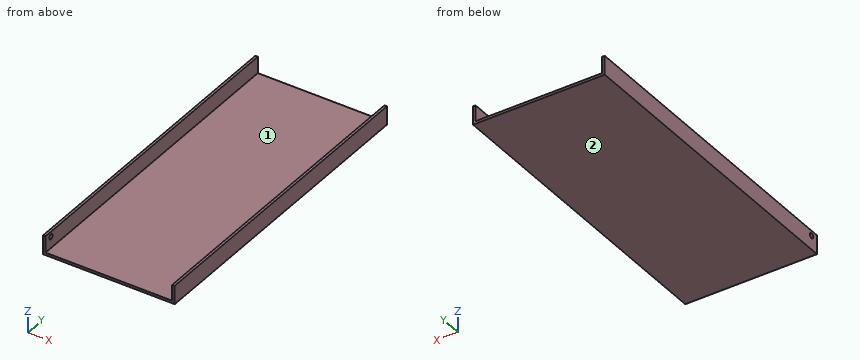
```python
from build123d import *

# Parameters (mm, degrees)
F1_DEPTH = 500
F3_D     = 8
F3_DEPTH = 12


with BuildPart() as f1:
    # F0 (on Front) → F1 (new body)
    with BuildSketch(Plane.XZ):
        Polygon((-104, 30), (-104, 0), (104, 0), (104, 29.331477), (100, 29.331477), (100, 4), (-100, 4), (-100, 30), align=None)
    extrude(amount=-F1_DEPTH)

    # F3
    with Locations(Plane(origin=(-104, 0, 0), x_dir=(0, -1, 0), z_dir=(-1, 0, 0))):
        with Locations((-12.759611, 22.157129)):
            Hole(F3_D / 2, depth=F3_DEPTH)


solid = f1.part
```
Geometry check sheet. Reference: the model listing, model coordinates, mm. Face numbers are marked on the shaded views. Coordinates: 2 decimals unless noted, no trailing zeros. Loops run counter-clockwise (first coordinate to the right, second up) from the corner with the lowest first, then second, coordinate; pieces in that order, holes last.
Item 1: Thickness scan on line 1 (X direction, y = 106, z = 25); line 2 (Z direction, x = -19, y = 406.5). Record the ranges inside material, lowest first.
Item 2: Sectioned sample at C-C, the plane x = 53. Record the boundary of the cut face in (y, z).
Item 3: Release check for a two-part mould opening along X. For the marked faces 1 and 2 record: released by +X, released by -X, zero draft, split by the parting line, or undercut.
Item 4: Sectioned sample at B-B, the plane y = 225.5. Record the boundary of the cut face in (x, z), then the cut area to 3 significant figures.
Item 5: Sectioned sample at A-A, the plane z = 12.25. Record the boundary of the cut face in (x, y).
Item 6: Go/stop test with flat-tipped pins: pin 1 Ø1.5 at (x, y) = (-66, 235.5) entering from +Z; pin 2 Ø1.2 at (x, y) = (101.5, 190) entering from +Z; pin 3 Ø3 at (x, y) = (-7.5, 162.5) entering from -Z. Record where each tip stops, or that it passes through.
Check result:
1. line 1: x = -104 to -100, 100 to 104
1. line 2: z = 0 to 4
2. outline: (0, 0) - (500, 0) - (500, 4) - (0, 4) - close
3. face 1: undercut
3. face 2: zero draft
4. outline: (-104, 0) - (104, 0) - (104, 29.33) - (100, 29.33) - (100, 4) - (-100, 4) - (-100, 30) - (-104, 30) - close
4. area: 1,040 mm2
5. outline: (-104, 0) - (-100, 0) - (-100, 500) - (-104, 500) - close; (100, 0) - (104, 0) - (104, 500) - (100, 500) - close
6. pin 1: stops at z = 4
6. pin 2: stops at z = 29.33
6. pin 3: stops at z = 0
